Geometry check sheet. Reference: the model listing, model coordinates, mm. Round coordinates to 2 decimals unless told otherwise and drop trailing zeros. Write each loop counter-clockwise with the first axis right and the second up, starting at its lowest first coordinate (ties: lowest second). Pieces come first, ordered by that corner, then holes. Notation, with made-up numbers: (-30.5, 5) - (0.5, 5) arc R13 ccw to (0.5, 10) - close; hole circle Ø9 at (14, 54.5). An arc over 180 degrees is marked (long way). Return JSON: item names as keys, results as strings.
Autodesk Inventor part; units mm, degrees
ref_plane "YZ Plane" through (0, 0, 0) normal (1, 0, 0) x (0, 1, 0)
ref_plane "XZ Plane" through (0, 0, 0) normal (0, 1, 0) x (-1, 0, 0)
ref_plane "XY Plane" through (0, 0, 0) normal (0, 0, 1) x (1, 0, 0)
sketch "Sketch1" plane through (0, 0, 0) normal (0, 0, 1) x (1, 0, 0)
  line L0 (4.6765, 0) -> (2.3383, -4.05)
  line L1 (2.3383, -4.05) -> (-2.3383, -4.05)
  line L2 (-2.3383, -4.05) -> (-4.6765, 0)
  line L3 (-4.6765, 0) -> (-2.3383, 4.05)
  line L4 (-2.3383, 4.05) -> (2.3383, 4.05)
  line L5 (2.3383, 4.05) -> (4.6765, 0)
  point P0 (0, 0)
  point P1 (0, 0)
  dimension "d0" = 8.1
extrude "Extrusion1" add sketch "Sketch1" along normal mid plane 2.1
sketch "Sketch2" plane through (0, 0, -1.05) normal (0, 0, -1) x (1, 0, 0)
  circle A0 centre (0, 0) radius 2.7
  dimension "d3" = 5.4
extrude "Extrusion2" cut sketch "Sketch2" against normal blind 2.1
fillet "Fillet2" radius 0.3 6 edges at (-2.3383, 4.05, 0) (2.3383, 4.05, 0) (-4.6765, 0, 0) (-2.3383, -4.05, 0) (2.3383, -4.05, 0) (4.6765, 0, 0)
sketch "Sketch4" plane through (0, 0, 0) normal (1, 0, 0) x (0, 1, 0)
  line L0 (2.7, 1.05) -> (5, 1.05)
  line L1 (5, 1.05) -> (5, 0.6444)
  line L2 (5, 0.6444) -> (2.7, 1.05)
  line L3 (-2.7, 1.05) -> (2.7, 1.05)
  line L4 (0, 6.5189) -> (0, -6.6611) construction
  line L5 (0, -9.297) -> (0, 9.1548)
  point P0 (0, 0)
  point P1 (5, 0.8472)
  dimension "d26" = 5
  dimension "d27" = 10
revolve "Revolution2" cut sketch "Sketch4" angle 360 about axis through (0, 0, 6.5189) along (0, 0, -1)
mirror "Mirror2" about plane through (0, 0, 0) normal (0, 0, 1) of "Revolution2"
chamfer "Chamfer4" distance 0.2 angle 45 4 edges at (-1.9092, -1.9092, 1.05) (1.9092, 1.9092, 1.05) (-1.9092, -1.9092, -1.05) (1.9092, 1.9092, -1.05)
properties part number "ecrou"
(1) Section check C-C, the plane y = 0. Enter the section's corners in (x, z).
Response values:
{"outline": "(-4.63, -0.71) - (-2.9, -1.02) - (-2.7, -0.85) - (-2.7, 0.85) - (-2.9, 1.02) - (-4.63, 0.71) - close; (2.7, -0.85) - (2.9, -1.02) - (4.63, -0.71) - (4.63, 0.71) - (2.9, 1.02) - (2.7, 0.85) - close"}
(2) Material ranges on line 1 along X through (y, z) = (0, -0.4); line 2 along Y through (x, z) = (0, -0.3); line 3 along Y through (x, z) = (-2.25, -0.2), recorded low to high. Write a range as [from, to].
Response values:
{"line 1": "x = [-4.63, -2.7], [2.7, 4.63]", "line 2": "y = [-4.05, -2.7], [2.7, 4.05]", "line 3": "y = [-4.04, -1.49], [1.49, 4.04]"}
(3) Section check B-B, the plane z = -0.15. Enter the section's corners in (x, y), plus the area to 3 significant figures.
Response values:
{"outline": "(-4.59, -0.15) - (-2.42, -3.9) arc R0.3 ccw to (-2.17, -4.05) - (2.17, -4.05) arc R0.3 ccw to (2.42, -3.9) - (4.59, -0.15) arc R0.3 ccw to (4.59, 0.15) - (2.42, 3.9) arc R0.3 ccw to (2.17, 4.05) - (-2.17, 4.05) arc R0.3 ccw to (-2.42, 3.9) - (-4.59, 0.15) arc R0.3 ccw to start; hole circle Ø5.4 at (0, 0)", "area": "33.9 mm^2"}
(4) Section check A-A, the plane x = 0. Enter the section's corners in (y, z), plus the area to 3 significant figures.
Response values:
{"outline": "(-4.05, -0.81) - (-2.9, -1.02) - (-2.7, -0.85) - (-2.7, 0.85) - (-2.9, 1.02) - (-4.05, 0.81) - close; (2.7, -0.85) - (2.9, -1.02) - (4.05, -0.81) - (4.05, 0.81) - (2.9, 1.02) - (2.7, 0.85) - close", "area": "4.95 mm^2"}
(5) Release check for a two-part mould opening along X. For faces 1 (the face through (-0.585, 2.636, -0.012)), 2 (the face through (3.492, 2.051, -0.011)), 3 (the face through (0, -4.05, 0)) record: pulls with the +X half, pulls with the -X half, needs draft (parallel to the pull), parting line crosses it, or undercut.
Response values:
{"face 1": "undercut", "face 2": "pulls with the +X half", "face 3": "needs draft"}
